from build123d import *

# Parameters (mm, degrees)
BOSS_EXTRUDE1_DEPTH     = 23
CUT_EXTRUDE2_DEPTH      = 23
CUT_EXTRUDE2_DEPTH_BACK = 10
SKETCH4_W               = 3.5
SKETCH4_H               = 21
SKETCH5_W               = 45
SKETCH5_H               = 7.5
CUT_EXTRUDE3_DEPTH      = 26
SKETCH7_R               = 1.45
CUT_EXTRUDE4_DEPTH      = 50
SKETCH8_W               = 13
SKETCH8_H               = 15.5
BOSS_EXTRUDE2_DEPTH     = 2.5
SKETCH9_R               = 1.45
CUT_EXTRUDE5_DEPTH      = 10
SKETCH10_W              = 15.5
SKETCH10_H              = 4
CUT_EXTRUDE7_DEPTH      = 6
SKETCH11_W              = 15.5
SKETCH11_H              = 4
CUT_EXTRUDE8_DEPTH      = 6


with BuildPart() as part:
    # Sketch1 → Boss-Extrude1 (new body)
    with BuildSketch(Plane.XY):
        with BuildLine():
            Line((0, 3), (0, 17))
            ThreePointArc((0, 17), (1.464466094, 20.535533906), (5, 22))
            Line((5, 22), (22, 22))
            ThreePointArc((22, 22), (25.535533906, 20.535533906), (27, 17))
            Line((27, 17), (27, 3))
            ThreePointArc((27, 3), (27.878679656, 0.878679656), (30, 0))
            Line((30, 0), (36, 0))
            Line((36, 0), (36, -4))
            Line((36, -4), (23, -4))
            Line((23, -4), (23, 18))
            Line((23, 18), (4, 18))
            Line((4, 18), (4, -4))
            Line((4, -4), (-9, -4))
            Line((-9, -4), (-9, 0))
            Line((-9, 0), (-3, 0))
            ThreePointArc((-3, 0), (-0.878679656, 0.878679656), (0, 3))
        make_face()
    extrude(amount=BOSS_EXTRUDE1_DEPTH)

    # Sketch4 → Cut-Extrude2 (cut, two sides: drawn at the far end of the back side and taken through both)
    with BuildSketch(Plane.ZY.offset(-CUT_EXTRUDE2_DEPTH_BACK)):
        with Locations((5.75, 6.5)):
            Rectangle(SKETCH4_W, SKETCH4_H)
    extrude(amount=CUT_EXTRUDE2_DEPTH + CUT_EXTRUDE2_DEPTH_BACK, mode=Mode.SUBTRACT)

    # Sketch5 → Cut-Extrude3 (cut)
    with BuildSketch(Plane(origin=(0, 22, 0), x_dir=(1, 0, 0), z_dir=(0, 1, 0))):
        with Locations((13.5, -3.75)):
            Rectangle(SKETCH5_W, SKETCH5_H)
    extrude(amount=-CUT_EXTRUDE3_DEPTH, mode=Mode.SUBTRACT)

    # Sketch7 → Cut-Extrude4 (cut)
    with BuildSketch(Plane(origin=(0, 0, 0), x_dir=(1, 0, 0), z_dir=(0, 1, 0))):
        with Locations(Location((-6, -15.25, 0), (0, 0, 270))):
            Circle(SKETCH7_R)
        with Locations(Location((33, -15.25, 0), (0, 0, 180))):
            Circle(SKETCH7_R)
    extrude(amount=-CUT_EXTRUDE4_DEPTH, mode=Mode.SUBTRACT)

    # Sketch8 → Boss-Extrude2 (add)
    with BuildSketch(Plane.XZ.offset(4)):
        with Locations((29.5, 15.25)):
            Rectangle(SKETCH8_W, SKETCH8_H)
        with Locations((-2.5, 15.25)):
            Rectangle(SKETCH8_W, SKETCH8_H)
    extrude(amount=BOSS_EXTRUDE2_DEPTH)

    # Sketch9 → Cut-Extrude5 (cut)
    with BuildSketch(Plane(origin=(0, -4, 0), x_dir=(1, 0, 0), z_dir=(0, 1, 0))):
        with Locations((33, -15.25)):
            Circle(SKETCH9_R)
        with Locations(Location((-6, -15.25, 0), (0, 0, 270))):
            Circle(SKETCH9_R)
    extrude(amount=-CUT_EXTRUDE5_DEPTH, mode=Mode.SUBTRACT)

    # Sketch10 → Cut-Extrude7 (cut)
    with BuildSketch(Plane.ZY.offset(9)):
        with Locations((15.25, -2)):
            Rectangle(SKETCH10_W, SKETCH10_H)
    extrude(amount=-CUT_EXTRUDE7_DEPTH, mode=Mode.SUBTRACT)

    # Sketch11 → Cut-Extrude8 (cut)
    with BuildSketch(Plane(origin=(36, 0, 0), x_dir=(0, 0, -1), z_dir=(1, 0, 0))):
        with Locations((-15.25, -2)):
            Rectangle(SKETCH11_W, SKETCH11_H)
    extrude(amount=-CUT_EXTRUDE8_DEPTH, mode=Mode.SUBTRACT)


solid = part.part
Input: part model. Units: mm. Frame: model coordinates. A direction names the side the tool comes from. Coordinates: 2 decimals unless noted, no trailing zeros. Order: outer loops, then holes, each group sorted by start corner. A loop starts at its lowest first (then second) coordinate and runs counter-clockwise, first axis right, second up. Notation, with made-up numbers: M 74,24.25 L 88,24.25 A27 cw 88,41.25 Z; hole C 81,49 d5. An arc over 180 degrees is marked long. Answer as CSV lines item,"result".
1. Access query for faces 1 (the flat face through (-3, -2, 15)), 2 (the flat face through (27, 10, 15)), 3 (the flat face through (29, -6.5, 15)), 4 (the flat face through (23, 6, 15)). Directions: +Z, -Z, +X, -X, +Y, -Y. A direction counts if a zero-diameter tool reaches every point of the face in a straight line with its end or side. Return the directions, or none.
Reported:
face 1,"+Z, -Z, -X, +Y"
face 2,"+Z, -Z, +X, +Y"
face 3,"+Z, -Z, +X, -X, -Y"
face 4,"+Z, -Z, -Y"
2. Section C-C (z = 15.25). Return the cut outline in (x, y), then the cut area to 3 significant figures.
Reported:
outline,"M -9,-6.5 L -7.45,-6.5 L -7.45,-4 L -9,-4 Z; M -4.55,-6.5 L 4,-6.5 L 4,18 L 23,18 L 23,-6.5 L 31.55,-6.5 L 31.55,-4 L 30,-4 L 30,0 A3 cw 27,3 L 27,17 A5 ccw 22,22 L 5,22 A5 ccw 0,17 L 0,3 A3 cw -3,0 L -3,-4 L -4.55,-4 Z; M 34.45,-6.5 L 36,-6.5 L 36,-4 L 34.45,-4 Z"
area,"352 mm2"
3. First-contact query: P1, Ø8, axis at y = 15, z = 17.5, coming from the -X side; P2, Ø10, axis at x = 15, y = 12, coming from the +Z side; P3, Ø7, axis at y = 7, z = 12.5, coming from the +X side; P4, Ø1.2, axis at y = -2.5, z = 13, coming from the +X side. Flat tips, straight axial feed; report the tip coordinate or a pass-through.
Reported:
P1,"x = 0"
P2,"through"
P3,"x = 27"
P4,"x = 30"
4. Section A-A (x = 33). Return the cut outline in (y, z), then the cut area to 3 significant figures.
Reported:
outline,"M -6.5,7.5 L -4,7.5 L -4,13.8 L -6.5,13.8 Z; M -6.5,16.7 L -4,16.7 L -4,23 L -6.5,23 Z"
area,"31.5 mm2"
5. Material intervals for line 1 (X direction, y = -5.95, z = 15.25); line 2 (X direction, y = 6.5, z = 12.25); line 3 (Z direction, x = 33, y = -5.05), sorted ascending. Write a range as from..to.
Reported:
line 1,"-9..-7.45, -4.55..4, 23..31.55, 34.45..36"
line 2,"0..4, 23..27"
line 3,"7.5..13.8, 16.7..23"
6. Section D-D (z = 20.75). Return the cut outline in (x, y).
Reported:
outline,"M -9,-6.5 L 4,-6.5 L 4,18 L 23,18 L 23,-6.5 L 36,-6.5 L 36,-4 L 30,-4 L 30,0 A3 cw 27,3 L 27,17 A5 ccw 22,22 L 5,22 A5 ccw 0,17 L 0,3 A3 cw -3,0 L -3,-4 L -9,-4 Z"
7. Pull-direction query (X, two-part tool) for faces 5 (the flat face through (14, 18, 15)), 6 (the cylindrical face through (34.38, -5.23, 14.81)), 7 (the cylindrical face through (-0.9, 0.86, 15.14)), 8 (the cylindrical face through (25, 21, 15)); classes: released by +X, released by -X, zero draft, split by the parting line, or undercut.
Reported:
face 5,"undercut"
face 6,"undercut"
face 7,"released by -X"
face 8,"released by +X"
8. Section B-B (y = 10.5). Return the cut outline in (x, z).
Reported:
outline,"M 0,7.5 L 4,7.5 L 4,23 L 0,23 Z; M 23,7.5 L 27,7.5 L 27,23 L 23,23 Z"
